The model under review builds one solid part; all positions refer to its coordinate system, in mm. Face numbers are marked on the shaded views. Round coordinates to 2 decimals unless told otherwise and drop trailing zeros. Order: outer loops, then holes, each group sorted by start corner. A loop starts at its lowest first (then second) coordinate and runs counter-clockwise, first axis right, second up.
1) Consider section C-C (x = 2). Give the boundary of the cut face in (y, z).
2) To check wall thickness, follow L1, parallel to Y at x = 0, z = 2.65; L2, parallel to Y at x = -0.75, z = 3.05; L3, parallel to X at y = -0.75, z = 0.9. State the ranges of each line that lie inside material, in increasing order.
3) Consider section B-B (y = 1.25). Give the boundary of the cut face in (x, z), then the cut area to 3 significant figures.
4) Consider section D-D (z = 3.8). Give the boundary of the cut face in (x, y), then the cut area to 3 significant figures.
5) Consider section A-A (x = 0). Give the boundary of the cut face in (y, z).
6) Mouldability with a two-part tool opening along Y and no side actions: class the marked faces 1, 2, 3 and 4 as pulls with the +Y half, pulls with the -Y half, needs draft (parallel to the pull), parting line crosses it, or undercut.
7) Clearance check with a flat-ended pin moving along its axis: P1, Ø2, axis at x = 1, y = -0.5, coming from the -Z side. State where the tip first meets the part, or that it passes through.
from build123d import *

# Parameters (mm, degrees)
CROQUIS1_R              = 2.5
CROQUIS1_R_2            = 0.5
SALIENTE_EXTRUIR1_DEPTH = 5


with BuildPart() as part:
    # Croquis1 → Saliente-Extruir1 (new body)
    with BuildSketch(Plane.XY):
        with BuildLine():
            Line((-3.5, 0), (-1.5, -16))
            ThreePointArc((-1.5, -16), (0, -17.5), (1.5, -16))
            Line((1.5, -16), (3.5, 0))
            ThreePointArc((3.5, 0), (0, 3.5), (-3.5, 0))
        make_face()
        Circle(CROQUIS1_R, mode=Mode.SUBTRACT)
        with Locations((0, -16)):
            Circle(CROQUIS1_R_2, mode=Mode.SUBTRACT)
    extrude(amount=SALIENTE_EXTRUIR1_DEPTH)


solid = part.part
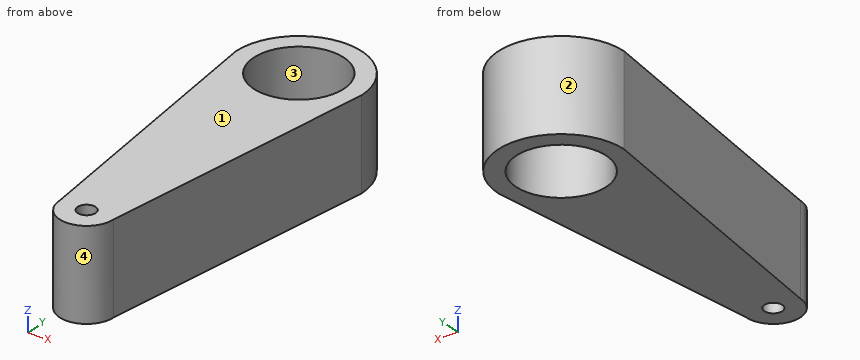
Answer below:
1. outline: (-12, 0) - (-1.5, 0) - (-1.5, 5) - (-12, 5) - close; (1.5, 0) - (2.87, 0) - (2.87, 5) - (1.5, 5) - close
2. L1: y = -17.5 to -16.5, -15.5 to -2.5, 2.5 to 3.5
2. L2: y = -17.3 to -2.38, 2.38 to 3.42
2. L3: x = -3.41 to -2.38, 2.38 to 3.41
3. outline: (-3.27, 0) - (-2.17, 0) - (-2.17, 5) - (-3.27, 5) - close; (2.17, 0) - (3.27, 0) - (3.27, 5) - (2.17, 5) - close
3. area: 11.0 mm2
4. outline: (-3.5, 0) - (-1.5, -16) arc R1.5 ccw to (1.5, -16) - (3.5, 0) arc R3.5 ccw to start; hole circle Ø5 at (0, 0); hole circle Ø1 at (0, -16)
4. area: 82.4 mm2
5. outline: (-17.5, 0) - (-16.5, 0) - (-16.5, 5) - (-17.5, 5) - close; (-15.5, 0) - (-2.5, 0) - (-2.5, 5) - (-15.5, 5) - close; (2.5, 0) - (3.5, 0) - (3.5, 5) - (2.5, 5) - close
6. face 1: needs draft
6. face 2: pulls with the +Y half
6. face 3: undercut
6. face 4: pulls with the -Y half
7. P1: passes through
